Geometry: final body of the model. Coordinates: model frame, mm. Coordinates: 2 decimals unless noted, no trailing zeros. Order: outer loops, then holes, each group sorted by start corner. A loop starts at its lowest first (then second) coordinate and runs counter-clockwise, first axis right, second up. Notation, with made-up numbers: M 14,65 L 67,65 A15 ccw 67,74 Z; hole C 65.5,32.5 d1. An arc over 180 degrees is marked long. Use CSV: the item, a comma, the result in double quotes. Start each with the question number.
Q1. Section query C-C, the plane y = 4.5. Output: boundary loops of the cut face in (x, z), and give its area (3 significant figures).
Q2. First-contact query: P1, Ø1, axis at y = 4, z = 3.5, coming from the +X side. Flat tip, straight axial feed; report the tip coordinate or a pass-through.
Q3. Section query A-A, the plane x = 0. Output: boundary loops of the cut face in (y, z), and give its area (3 significant figures).
Q4. Ray query, probe 1 along Z at (x, y) = (0, 1.85); probe 2 along X at (y, z) = (0.5, -1); probe 3 along X at (y, z) = (1.2, -2.5). Return the intervals inside material, ascending.
Q5. Mould query, pull axis Z, two halves, no side actions, for faces 1 (the face through (0, 0, -7)), 2 (the face through (0, 2, 10)), 3 (the face through (0, 2, -18)), 4 (the face through (5, 2.5, 1.6)). Classes: +Z half, -Z half, draft (parallel to the pull), parting line (faces both ways), or undercut.
Q6. Section query D-D, the plane z = 8. Output: boundary loops of the cut face in (x, y), and give its area (3 significant figures).
Q7. Section query B-B, the plane z = 2. Output: boundary loops of the cut face in (x, y).
from build123d import *

# Parameters (mm, degrees)
F0_R     = 5.25
F1_DEPTH = 5


with BuildPart() as f1:
    # F0 (on Front) → F1 (new body)
    with BuildSketch(Plane.XZ):
        with BuildLine():
            Line((10, -18), (10, 0))
            ThreePointArc((10, 0), (0, -10), (-10, 0))
            Line((-10, 0), (-10, -18))
            Line((-10, -18), (10, -18))
        make_face()
        with BuildLine():
            ThreePointArc((-10, 0), (0, -10), (10, 0))
            ThreePointArc((10, 0), (0, 10), (-10, 0))
        make_face()
        Circle(F0_R, mode=Mode.SUBTRACT)
    extrude(amount=-F1_DEPTH)


solid = f1.part
Responses:
1,outline,"M -10,-18 L 10,-18 L 10,0 A10 ccw -10,0 Z; hole C 0,0 d10.5"
1,area,"430 mm²"
2,P1,"stops at x = 9.54"
3,outline,"M 0,-18 L 5,-18 L 5,-5.25 L 0,-5.25 Z; M 0,5.25 L 5,5.25 L 5,10 L 0,10 Z"
3,area,"87.5 mm²"
4,probe 1,"z = -18 to -5.25, 5.25 to 10"
4,probe 2,"x = -10 to -5.15, 5.15 to 10"
4,probe 3,"x = -10 to -4.62, 4.62 to 10"
5,face 1,"draft"
5,face 2,"+Z half"
5,face 3,"-Z half"
5,face 4,"undercut"
6,outline,"M -6,0 L 6,0 L 6,5 L -6,5 Z"
6,area,"60.0 mm²"
7,outline,"M -9.8,0 L -4.85,0 L -4.85,5 L -9.8,5 Z; M 4.85,0 L 9.8,0 L 9.8,5 L 4.85,5 Z"
